The drawing under review shows one solid part. Ordinate dimensions are in mm from its lowest x, y, z. Give positions to 0.01 mm unless a question says otherwise; leave off trailing zeros. Loops run counter-clockwise (first coordinate to the right, second up) from the corner with the lowest first, then second, coordinate; pieces in that order, holes last.
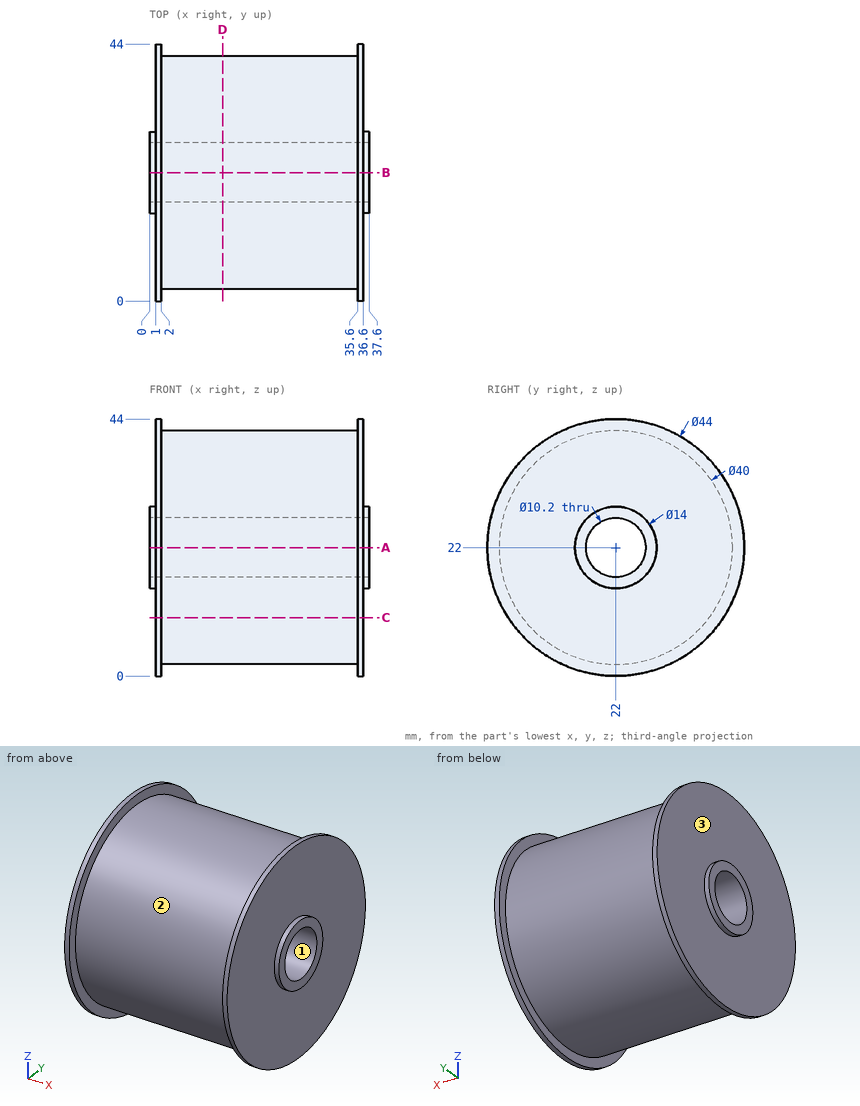
Item 1: The part is to be moulded in two halves that separate along X. For the marked faces 1, 2 and 3, say which applies: released by +X, released by -X, zero draft, split by the parting line, or undercut.
Answer:
face 1: zero draft
face 2: undercut
face 3: released by -X
Item 2: Take a section at C-C on z = 10. Give the boundary of the cut face in (x, y), and give its area (3 significant figures).
Answer:
outline: (1, 3.56) - (2, 3.56) - (2, 6) - (35.6, 6) - (35.6, 3.56) - (36.6, 3.56) - (36.6, 40.44) - (35.6, 40.44) - (35.6, 38) - (2, 38) - (2, 40.44) - (1, 40.44) - close
area: 1,150 mm2
Item 3: Take a section at A-A on z = 22. Give the boundary of the cut face in (x, y), and give its area (3 significant figures).
Answer:
outline: (0, 15) - (1, 15) - (1, 0) - (2, 0) - (2, 2) - (35.6, 2) - (35.6, 0) - (36.6, 0) - (36.6, 15) - (37.6, 15) - (37.6, 16.9) - (0, 16.9) - close; (0, 27.1) - (37.6, 27.1) - (37.6, 29) - (36.6, 29) - (36.6, 44) - (35.6, 44) - (35.6, 42) - (2, 42) - (2, 44) - (1, 44) - (1, 29) - (0, 29) - close
area: 1,080 mm2
Item 4: Clearance check with flat-ended pins moving along their axes: pin 1 Ø9 at (y, z) = (22, 22) entering from +X; pin 2 Ø4 at (x, z) = (32, 6.5) entering from -Y; pin 3 Ø12 at (y, z) = (5, 22) entering from -X; pin 4 Ø10 at (x, z) = (7.5, 15) entering from +Y. State where each tip first meets the part, or that it passes through.
Answer:
pin 1: passes through
pin 2: stops at y = 7.24
pin 3: stops at x = 1
pin 4: stops at y = 41.9
Item 5: Take a section at D-D on x = 12.5. Give the boundary of the cut face in (y, z).
Answer:
outline: circle Ø40 at (22, 22); hole circle Ø10.2 at (22, 22)
Item 6: For L1, parallel to Z at x = 24, y = 22; L2, parallel to X at y = 29.5, z = 5.5; L3, parallel to X at y = 4, z = 11.5, list the stretches that pass through material, from the lowest coordinate up.
Answer:
L1: z = 2 to 16.9, 27.1 to 42
L2: x = 1 to 36.6
L3: x = 1 to 2, 35.6 to 36.6
